Read the model definition and answer for the solid it produces. Units are mm, in the model's axes. Give positions to 0.01 mm unless a question says otherwise; leave off trailing zeros. Write each loop counter-clockwise with the first axis right and the second up, starting at its lowest first coordinate (ties: lowest second). Pieces come first, ordered by that corner, then holes. Notation, with made-up numbers: M -14,31.5 L 0,31.5 A20 cw 0,68.5 Z; hole C 25,1.25 d1. An arc over 180 degrees is marked long. Use a Markdown table: item, result. Add a question column.
Item 1: Given P1, Ø2, axis at x = 37, y = -1, coming from the -Z side; P2, Ø6, axis at y = 0, z = -114.5, coming from the -X side; P3, Ø2, axis at x = 80.5, y = 8, coming from the -Z side, each flat-ended and moving along its own axis, determine where each tip first touches the part or whether it passes through.
Item 2: A cutting plane is placed at B-B on z = -143. Determine the outline of the cut face in (x, y).
Item 3: Consider probe 1 along Z at (x, y) = (-9.5, -0.75); probe 2 along Z at (x, y) = (5, 10.5); probe 3 along Z at (x, y) = (8, 7.75). Determine where each line is inside the solid, lowest interval first. Write a range as [from, to].
Item 4: A cutting plane is placed at C-C on x = 32.5. Determine the outline of the cut face in (y, z).
Item 5: A cutting plane is placed at A-A on y = 6.5. Determine the outline of the cut face in (x, z), then the cut area to 3 significant figures.
from build123d import *

# Parameters (mm, degrees)
BOSS_EXTRUDE1_DEPTH = 12
BOSS_EXTRUDE2_DEPTH = 2
BOSS_EXTRUDE3_DEPTH = 2


with BuildPart() as part:
    # Sketch1 → Boss-Extrude1 (new body)
    with BuildSketch(Plane(origin=(0, 0, 0), x_dir=(1, 0, 0), z_dir=(0, 1, 0))):
        Polygon((109.556624327, -4.42820323), (-109.556624327, -4.42820323), (-112.113248654, 0), (-2.556624327, 189.75763964), (2.556624326, 189.75763964), (112.113248654, 0), align=None)
        Polygon((-107.82457352, -1.42820323), (-108.649147039, 0), (-99.473720558, 15.892304845), (-89.473720558, -1.42820323), align=None, mode=Mode.SUBTRACT)
        Polygon((-0.82457352, 186.75763964), (0.824573518, 186.75763964), (9.999999999, 170.865334794), (-10.000000001, 170.865334794), align=None, mode=Mode.SUBTRACT)
        Polygon((108.649147039, 0), (107.82457352, -1.42820323), (89.473720559, -1.42820323), (99.473720559, 15.892304846), align=None, mode=Mode.SUBTRACT)
        Polygon((-11.732050808, 167.865334795), (11.732050808, 167.865334795), (97.741669751, 18.892304846), (86.009618944, -1.42820323), (-86.009618943, -1.42820323), (-97.741669751, 18.892304845), align=None, mode=Mode.SUBTRACT)
    extrude(amount=BOSS_EXTRUDE1_DEPTH)

    # Sketch1<4> → Boss-Extrude2 (add)
    with BuildSketch(Plane(origin=(0, 0, 0), x_dir=(1, 0, 0), z_dir=(0, 1, 0))):
        Polygon((11.732050808, 167.865334795), (-11.732050808, 167.865334795), (-97.741669751, 18.892304845), (-86.009618943, -1.42820323), (86.009618944, -1.42820323), (97.741669751, 18.892304846), align=None)
        with BuildLine():
            Line((-85.56624327, 2.803847577), (-93.854918405, 17.160254038))
            ThreePointArc((-93.854918405, 17.160254038), (-82.532377607, 14.126388375), (-85.56624327, 2.803847577))
        make_face(mode=Mode.SUBTRACT)
        with BuildLine():
            Line((84.566243271, 1.07179677), (-84.56624327, 1.07179677))
            ThreePointArc((-84.56624327, 1.07179677), (-80.800326799, 15.126388375), (-94.854918405, 18.892304845))
            Line((-94.854918405, 18.892304845), (-10.288675135, 165.365334795))
            Line((-10.288675135, 165.365334795), (10.288675135, 165.365334795))
            Line((10.288675135, 165.365334795), (94.854918405, 18.892304846))
            Line((94.854918405, 18.892304846), (84.566243271, 1.07179677))
        make_face(mode=Mode.SUBTRACT)
    extrude(amount=BOSS_EXTRUDE2_DEPTH)

    # Sketch2 → Boss-Extrude3 (add)
    with BuildSketch(Plane.XZ):
        Polygon((-87.741669751, 4.42820323), (-101.205771366, -18.892304846), (-99.473720559, -21.892304845), (-84.277568136, 4.42820323), align=None)
        Polygon((87.741669751, 4.42820323), (-74.277568136, 4.42820323), (-76.009618943, 1.42820323), (86.009618943, 1.42820323), (97.74166975, -18.892304845), (11.732050807, -167.865334795), (-11.732050808, -167.865334795), (-92.741669751, -27.552558883), (-94.473720559, -30.552558883), (-13.464101616, -170.865334794), (13.464101615, -170.865334794), (101.205771366, -18.892304845), align=None)
    extrude(amount=BOSS_EXTRUDE3_DEPTH)


solid = part.part
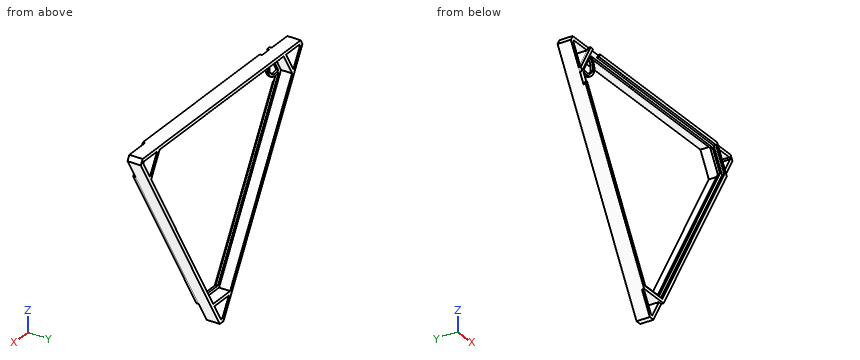
Filled in:
| question | item | result |
|---|---|---|
| 1 | P1 | z = -131.83 |
| 1 | P2 | x = -47.74 |
| 1 | P3 | z = -56.49 |
| 2 | outline | M -29.55,-2 L -26.09,-2 L -26.09,0 L -23.2,0 L -23.2,2 L -26.09,2 L -26.09,12 L -29.55,12 Z; M 23.2,0 L 26.09,0 L 26.09,-2 L 29.55,-2 L 29.55,12 L 26.09,12 L 26.09,2 L 23.2,2 Z |
| 3 | probe 1 | [-170.87, -167.87], [1.43, 4.43] |
| 3 | probe 2 | [-185.53, -179.53], [-170.87, -167.87], [1.43, 4.43] |
| 3 | probe 3 | [-180.33, -174.33], [-170.87, -167.87], [1.43, 4.43] |
| 4 | outline | M -2,-137.89 L 12,-137.89 L 12,-131.89 L 2,-131.89 L 2,-126.89 L 0,-126.89 L 0,-131.89 L -2,-131.89 Z; M -2,1.43 L 0,1.43 L 0,-1.07 L 2,-1.07 L 2,1.43 L 12,1.43 L 12,4.43 L -2,4.43 Z |
| 5 | outline | M -112.11,0 L -2.56,-189.76 L 2.56,-189.76 L 112.11,0 L 109.56,4.43 L -109.56,4.43 Z; hole M -108.65,0 L -99.47,-15.89 L -89.47,1.43 L -107.82,1.43 Z; hole M -97.74,-18.89 L -11.73,-167.87 L 11.73,-167.87 L 97.74,-18.89 L 86.01,1.43 L -86.01,1.43 Z; hole M -10,-170.87 L -0.82,-186.76 L 0.82,-186.76 L 10,-170.87 Z; hole M 89.47,1.43 L 99.47,-15.89 L 108.65,0 L 107.82,1.43 Z |
| 5 | area | 2,180 mm² |
